Design review of the part built by this model. Coordinates are the model's own, in mm. A direction names the side the tool comes from. Coordinates: 2 decimals unless noted, no trailing zeros. Loops run counter-clockwise (first coordinate to the right, second up) from the corner with the lowest first, then second, coordinate; pieces in that order, holes last. Notation, with made-up numbers: (81.5, -27) - (119.5, -27) arc R13 cw to (119.5, -23) - close; hole circle Ø4 at (19, 70.5). An arc over 180 degrees is marked (long way). Return JSON: item names as keys, results as strings. Group by question number.
from build123d import *

# Parameters (mm, degrees)
F0_W         = 5
F0_H         = 10
F0_R         = 1.75
F0_R_2       = 4
F0_R_3       = 11.5
F0_W_2       = 7.5
F0_H_2       = 8
F1_DEPTH     = 8
F3_DEPTH     = 30
F4_W         = 5
F4_H         = 15
F4_W_2       = 63
F4_R         = 4
F5_DEPTH     = 5
F6_R         = 4
F7_DEPTH     = 23
F9_DEPTH     = 73
F10_R        = 4
F11_R        = 2
F12_T1_DEPTH = 33


# Not quite as in the source:
# - a fillet or chamfer that OpenCascade refuses, or shapes differently, is made with other operations: its cross-section is extruded or revolved along the edge and cut away or added


with BuildPart() as f1:
    # F0 (on Top) → F1 (new body)
    with BuildSketch(Plane.XY):
        Polygon((0, 57), (0, 0), (22.5, 0), (30, 0), (37.25, 0), (37.25, 4), (36, 4), (36, 7), (37.25, 7), (37.25, 12), (40.75, 12), (40.75, 7), (42, 7), (42, 4), (40.75, 4), (40.75, 0), (48, 0), (55.5, 0), (73, 0), (73, 57), align=None)
        with Locations((7.5, 15.5)):
            Rectangle(F0_W, F0_H, mode=Mode.SUBTRACT)
        with Locations((23, 19.5)):
            Circle(F0_R, mode=Mode.SUBTRACT)
        with Locations((54, 19.5)):
            Circle(F0_R, mode=Mode.SUBTRACT)
        with Locations((65.5, 15.5)):
            Rectangle(F0_W, F0_H, mode=Mode.SUBTRACT)
        with Locations((7.5, 25.25)):
            Circle(F0_R, mode=Mode.SUBTRACT)
        with Locations((7.5, 35)):
            Rectangle(F0_W, F0_H, mode=Mode.SUBTRACT)
        with Locations((17, 35)):
            Circle(F0_R_2, mode=Mode.SUBTRACT)
        with Locations((23, 50.5)):
            Circle(F0_R, mode=Mode.SUBTRACT)
        with Locations((38.5, 35)):
            Circle(F0_R_3, mode=Mode.SUBTRACT)
        with Locations((65.5, 25.25)):
            Circle(F0_R, mode=Mode.SUBTRACT)
        with Locations((65.5, 35)):
            Rectangle(F0_W, F0_H, mode=Mode.SUBTRACT)
        with Locations((54, 50.5)):
            Circle(F0_R, mode=Mode.SUBTRACT)
        with Locations((51.75, -4)):
            Rectangle(F0_W_2, F0_H_2)
        with Locations((26.25, -4)):
            Rectangle(F0_W_2, F0_H_2)
    extrude(amount=-F1_DEPTH)

    # F2 (on Top) → F3 (join)
    with BuildSketch(Plane.XY):
        Polygon((0, 57), (0, 0), (5, 0), (5, 10.5), (5, 20.5), (5, 30), (5, 40), (5, 57), align=None)
        Polygon((73, 57), (68, 57), (68, 40), (68, 30), (68, 20.5), (68, 10.5), (68, 0), (73, 0), align=None)
    extrude(amount=F3_DEPTH)

    # F4 (on face) → F5 (join)
    with BuildSketch(Plane.XY.offset(30)):
        with Locations((2.5, 35.5)):
            Rectangle(F4_W, F4_H)
        with Locations((36.5, 35.5)):
            Rectangle(F4_W_2, F4_H)
        with Locations((17, 35)):
            Circle(F4_R, mode=Mode.SUBTRACT)
        with Locations((38.5, 35)):
            Circle(F4_R, mode=Mode.SUBTRACT)
        with Locations((70.5, 35.5)):
            Rectangle(F4_W, F4_H)
    extrude(amount=F5_DEPTH)

    # F6 (on face) → F7 (join)
    with BuildSketch(Plane.XY.offset(35)):
        with BuildLine():
            ThreePointArc((25, 35), (22.6568542495, 40.6568542495), (17, 43))
            ThreePointArc((17, 43), (9.2540333076, 37), (13.1270166538, 28))
            Line((13.1270166538, 28), (20.8729833462, 28))
            ThreePointArc((20.8729833462, 28), (23.8914391374, 30.9369879873), (25, 35))
        make_face()
        with Locations((17, 35)):
            Circle(F6_R, mode=Mode.SUBTRACT)
        with BuildLine():
            ThreePointArc((46.5, 35), (44.1568542495, 40.6568542495), (38.5, 43))
            ThreePointArc((38.5, 43), (30.7540333076, 37), (34.6270166538, 28))
            Line((34.6270166538, 28), (42.3729833462, 28))
            ThreePointArc((42.3729833462, 28), (45.3914391374, 30.9369879873), (46.5, 35))
        make_face()
        with Locations((38.5, 35)):
            Circle(F6_R, mode=Mode.SUBTRACT)
    extrude(amount=F7_DEPTH)

    # F8 (on face) → F9 (cut)
    with BuildSketch(Plane(origin=(0, 0, 0), x_dir=(0, -1, 0), z_dir=(-1, 0, 0))):
        Polygon((-57, 0), (-43, 30), (-57, 30), align=None)
        Polygon((0, 30), (-28, 30), (0, 0), align=None)
    extrude(amount=-F9_DEPTH, mode=Mode.SUBTRACT)

    # F10
    f10_edges = [f1.edges().sort_by_distance(p)[0] for p in [
        (0, 57, -4),
        (73, 57, -4),
        (0, 0, -4),
        (73, 0, -4),
    ]]
    fillet(f10_edges, radius=F10_R)

    # F11
    f11_edges = [f1.edges().sort_by_distance(p)[0] for p in [
        (73, 28, 32.5),
        (0, 28, 32.5),
        (0, 43, 32.5),
        (73, 43, 32.5),
    ]]
    fillet(f11_edges, radius=F11_R)

    # F12: fillet of radius 5 on 4 edges, made by hand

    # F12_s2 → F12_t1 (cut)
    with BuildSketch(Plane.XY.offset(-20.5)):
        with BuildLine():
            ThreePointArc((25, -8), (28.5355339059, -6.5355339059), (30, -3))
            Line((30, -3), (30, -8))
            Line((30, -8), (25, -8))
        make_face()
        with BuildLine():
            ThreePointArc((22.5, -3), (23.9644660941, -6.5355339059), (27.5, -8))
            Line((27.5, -8), (22.5, -8))
            Line((22.5, -8), (22.5, -3))
        make_face()
        with BuildLine():
            ThreePointArc((55.5, -3), (54.0355339059, -6.5355339059), (50.5, -8))
            Line((50.5, -8), (55.5, -8))
            Line((55.5, -8), (55.5, -3))
        make_face()
        with BuildLine():
            ThreePointArc((53, -8), (49.4644660941, -6.5355339059), (48, -3))
            Line((48, -3), (48, -8))
            Line((48, -8), (53, -8))
        make_face()
    extrude(amount=F12_T1_DEPTH, mode=Mode.SUBTRACT)


with BuildPart() as f13_1:
    # F13: instance of F1
    add(f1.part.mirror(Plane(origin=(0, 30.6667140421, 8.8934527193), x_dir=(0, -1, 0), z_dir=(-1, 0, 0))))


solid = f13_1.part
Item 1: Add section A-A (x = -7.5). State the section outline as (y, z) points, then the cut area to 3 significant figures.
Item 2: To check wall thickness, follow line 1 (Y direction, x = -7.5, z = -4.25); line 2 (X direction, y = 24.5, z = 8.5); line 3 (Y direction, x = -17, z = -5). State the ranges of each line that lie inside material, in increasing order. Write a range as from..to.
Item 3: Draft analysis for pull direction X (two halves, no side actions). For faces 6 (the face through (-65, 30, -4)), 7 (the face through (-0.87, 42.65, 33.09)), 8 (the face through (-37, 57, -4)), state which applies: pulls with the +X half, pulls with the -X half, needs draft (parallel to the pull), parting line crosses it, or undercut.
Item 4: Add section D-D (z = 7). State the section outline as (x, y) points.
Item 5: Add section C-C (y = 50.5). State the section outline as (x, z) points.
Item 6: For faces 1 (the face through (-54.5, -6, -4.1)), 2 (the face through (-63, 15, -4)), 3 (the face through (-37, 43, 32)), 4 (the face through (-49, -6, -4)), 5 (the face through (-72.43, 28.6, 33.09)), list the 3-axis set-ups (+Z, -Z, +X, -X, +Y, -Y) from which the entire face can be reached by the end or side of a thin tool; tool diameter is ignored.
Item 7: Add section B-B (z = 37). State the section outline as (x, y) points.
Item 8: For P1, Ø12, axis at x = -16.5, z = 13, coming from the -Y side; P2, Ø1, axis at x = -37, z = -5.5, coming from the -Y side; P3, Ø22.5, axis at x = -49.5, z = 41, coming from the -Y side; P4, Ø0.9, axis at y = -1.5, z = -3.5, coming from the +X side, all flat-tipped, find the tip position at first contact; note any pin that passes through.
Answers below:
{
 "1": {"outline": "(0, -8) - (10.5, -8) - (10.5, 0) - (0, 0) - close; (20.5, -8) - (23.5, -8) - (23.5, 0) - (20.5, 0) - close; (27, -8) - (30, -8) - (30, 0) - (27, 0) - close; (28, 30) - (43, 30) - (43, 35) - (28, 35) - close; (40, -8) - (57, -8) - (57, 0) - (40, 0) - close", "area": "343 mm^2"},
 "2": {"line 1": "y = 0..10.5, 20.5..23.5, 27..30, 40..57", "line 2": "x = -73..-68, -5..0", "line 3": "y = 0..31, 39..57"},
 "3": {"face 6": "undercut", "face 7": "pulls with the +X half", "face 8": "needs draft"},
 "4": {"outline": "(-73, 6.53) - (-68, 6.53) - (-68, 53.73) - (-72.93, 53.73) arc R4 ccw to (-73, 53) - close; (-5, 6.53) - (0, 6.53) - (0, 53) arc R4 ccw to (-0.07, 53.73) - (-5, 53.73) - close"},
 "5": {"outline": "(-73, -8) - (-55.75, -8) - (-55.75, 0) - (-68, 0) - (-68, 13.93) - (-73, 13.93) - close; (-52.25, -8) - (-24.75, -8) - (-24.75, 0) - (-52.25, 0) - close; (-21.25, -8) - (0, -8) - (0, 13.93) - (-5, 13.93) - (-5, 0) - (-21.25, 0) - close"},
 "6": {"face 1": "+Z, -Z, -X, -Y", "face 2": "+Z, -Z", "face 3": "+Z, +X, -X, +Y", "face 4": "+Z, -Z, -Y", "face 5": "+Z, -X, -Y"},
 "7": {"outline": "(-42.37, 28) - (-34.63, 28) arc R8 ccw (long way) to start; (-20.87, 28) - (-13.13, 28) arc R8 ccw (long way) to start; hole circle Ø8 at (-38.5, 35); hole circle Ø8 at (-17, 35)"},
 "8": {"P1": "passes through", "P2": "stops at y = 0", "P3": "stops at y = 28", "P4": "stops at x = -22.5"}
}
